from build123d import *

# Parameters (mm, degrees)
F1_DEPTH = 63.5
F2_DEPTH = 25.4
F3_DEPTH = 7.9375
F5_R     = 6.35


with BuildPart() as f1:
    # F0 (on Front) → F1 (new body, symmetric)
    with BuildSketch(Plane.XZ):
        Polygon((-41.275, 9.525), (-41.275, -9.525), (41.275, -9.525), (41.275, 9.525), (22.225, 9.525), align=None)
    extrude(amount=F1_DEPTH, both=True)

    # F0 (on Front) → F2 (join, symmetric)
    with BuildSketch(Plane.XZ):
        with BuildLine():
            Line((22.225, 9.525), (41.275, 9.525))
            Line((41.275, 9.525), (41.275, 27.0002))
            ThreePointArc((41.275, 27.0002), (45.92468, 38.22552), (57.15, 42.8752))
            Line((57.15, 42.8752), (60.325, 42.8752))
            Line((60.325, 42.8752), (60.325, 61.9252))
            Line((60.325, 61.9252), (57.15, 61.9252))
            add(Edge.make_bspline(
                [(55.738204, 61.896653), (56.207698, 61.907946), (56.678301, 61.917467), (57.15, 61.9252)],
                knots=[110.584211, 110.584211, 110.584211, 110.584211, 111.504536, 111.504536, 111.504536, 111.504536], degree=3))
            ThreePointArc((55.738204, 61.896653), (31.960095, 51.19161), (22.225, 27.0002))
            Line((22.225, 27.0002), (22.225, 9.525))
        make_face()
        Polygon((85.725, 61.9252), (60.325, 61.9252), (60.325, 42.8752), (85.725, 42.8752), (85.725, 52.3875), align=None)
    extrude(amount=F2_DEPTH, both=True)

    # F0 (on Front) → F3 (join, symmetric)
    with BuildSketch(Plane.XZ):
        with BuildLine():
            add(Edge.make_bspline(
                [(-41.275, 9.525), (-41.068148, 33.600268), (-0.675116, 60.539722), (55.738204, 61.896653)],
                knots=[0, 0, 0, 0, 110.584211, 110.584211, 110.584211, 110.584211], degree=3))
            Line((-41.275, 9.525), (22.225, 9.525))
            Line((22.225, 9.525), (22.225, 27.0002))
            ThreePointArc((22.225, 27.0002), (31.960095, 51.19161), (55.738204, 61.896653))
        make_face()
    extrude(amount=F3_DEPTH, both=True)

    # F0 (on Front) → F4 (revolve)
    with BuildSketch(Plane.XZ):
        Polygon((85.725, 66.675), (85.725, 61.9252), (85.725, 52.3875), (85.725, 42.8752), (85.725, 38.1), (111.125, 38.1), (111.125, 66.675), align=None)
    revolve(axis=Axis((85.725, 0, 57.15635), (0, 0, 1)))

    # F5
    f5_edges = [f1.edges().sort_by_distance(p)[0] for p in [
        (41.275, 63.5, 0),
        (-41.275, 63.5, 0),
        (41.275, -63.5, 0),
        (-41.275, -63.5, 0),
    ]]
    fillet(f5_edges, radius=F5_R)


solid = f1.part
Work out the finished part from the listing and answer in its coordinate system (mm). A direction names the side the tool comes from. Round coordinates to 2 decimals unless told otherwise and drop trailing zeros. Write each loop counter-clockwise with the first axis right and the second up, starting at its lowest first coordinate (ties: lowest second). Pieces come first, ordered by that corner, then holes. Notation, with made-up numbers: M 75,-22.75 L 128,-22.75 A20 cw 128,-17.75 Z; hole C 30,48 d8. An arc over 180 degrees is marked long. Use a Markdown table: item, result.
1) Consider line 1 (Y direction, x = 15, z = 30); line 2 (Z direction, x = 14.5, y = 44) (3 decimals); line 3 (X direction, y = -7, z = 9) (3 decimals). Determine where each line is inside the solid, lowest interval first. Write a range as [from, to].
Taken from the geometry:
| item | result |
|---|---|
| line 1 | y = [-7.94, 7.94] |
| line 2 | z = [-9.525, 9.525] |
| line 3 | x = [-41.275, 41.275] |
2) Determine the mould class of faces 5 (the face through (-1, -1, -9.525)), 6 (the face through (45.8, -0.4, 38.1)), 7 (the face through (22.225, 17, 18)) for opening direction X: pulls with the +X half, pulls with the -X half, needs draft (parallel to the pull), parting line crosses it, or undercut.
Taken from the geometry:
| item | result |
|---|---|
| face 5 | needs draft |
| face 6 | undercut |
| face 7 | pulls with the -X half |
3) The part is cut by section B-B on y = 39. Give the vertices of the cut face in (x, z) (3 decimals).
Taken from the geometry:
| item | result |
|---|---|
| outline | M -41.275,-9.525 L 41.275,-9.525 L 41.275,9.525 L -41.275,9.525 Z |
4) Flat-ended cylindrical pins translate along their axes: pin 1 (4 mm diameter, centred on x = 62, y = 0.5, fed in from -Z); pin 2 (6 mm diameter, centred on y = 17.5, z = 40, fed in from +X); pin 3 (5 mm diameter, centred on x = 45, y = -26.5, fed in from -Z). Find the tip coordinate at first contact, or state that the pin passes through.
Taken from the geometry:
| item | result |
|---|---|
| pin 1 | stops at z = 38.1 |
| pin 2 | stops at x = 106.58 |
| pin 3 | stops at z = 33.69 |
5) The part is cut by section A-A on z = 1.5. Give the vertices of the cut face in (x, y) (3 decimals).
Taken from the geometry:
| item | result |
|---|---|
| outline | M -41.275,-57.15 A6.35 ccw -34.925,-63.5 L 34.925,-63.5 A6.35 ccw 41.275,-57.15 L 41.275,57.15 A6.35 ccw 34.925,63.5 L -34.925,63.5 A6.35 ccw -41.275,57.15 Z |
6) Which of the six approach directions +Z, -Z, +X, -X, +Y, -Y give full straight-line access (tool end or side, diameter ignored) to faces 1 (the face through (-3, -7.938, 30)), 2 (the face through (1, 35, 9.525)), 3 (the face through (86, 0, 38.1)), 4 (the face through (46, 25.4, 42))?
Taken from the geometry:
| item | result |
|---|---|
| face 1 | +Z, -X, -Y |
| face 2 | +Z, -X, +Y |
| face 3 | -Z, +X, +Y, -Y |
| face 4 | +Z, +X, -X, +Y |
7) The part is cut by section C-C on x = 88.5. Give the vertices of the cut face in (y, z) (3 decimals).
Taken from the geometry:
| item | result |
|---|---|
| outline | M -25.248,38.1 L 25.248,38.1 L 25.248,66.675 L -25.248,66.675 Z |
